from build123d import *

# Parameters (mm, degrees)
SKETCH1_R                       = 8
BOSS_EXTRUDE1_DEPTH             = 10
SKETCH2_R                       = 12.6
BOSS_EXTRUDE2_DEPTH             = 3
SKETCH4_R                       = 1.5
CUT_EXTRUDE4_DEPTH              = 13
SKETCH3_R                       = 12.6
BOSS_EXTRUDE4_DEPTH             = 5
SKETCH5_R                       = 2.1
CUT_EXTRUDE5_DEPTH              = 19
SKETCH6_W                       = 1
SKETCH6_H                       = 4.89371283
BOSS_EXTRUDE5_DEPTH             = 8
TAP_DRILL_FOR_M2X0_4_TAP1_D     = 1.6
TAP_DRILL_FOR_M2X0_4_TAP1_DEPTH = 16
TAP_DRILL_FOR_M2X0_4_TAP1_TIP   = 0.480688495
SKETCH16_R                      = 15.644014
BOSS_EXTRUDE6_DEPTH             = 5
SKETCH17_R                      = 2.1
CUT_EXTRUDE6_DEPTH              = 5
SKETCH18_R                      = 1.1
CUT_EXTRUDE9_DEPTH              = 9.0000001
SKETCH19_R                      = 1.1
CUT_EXTRUDE10_DEPTH             = 10


with BuildPart() as part:
    # Sketch1 → Boss-Extrude1 (new body)
    with BuildSketch(Plane(origin=(0, 0, 0), x_dir=(1, 0, 0), z_dir=(0, 1, 0))):
        Circle(SKETCH1_R)
    extrude(amount=BOSS_EXTRUDE1_DEPTH)

    # Sketch2 → Boss-Extrude2 (add)
    with BuildSketch(Plane.XZ):
        Circle(SKETCH2_R)
    extrude(amount=BOSS_EXTRUDE2_DEPTH)

    # Sketch4 → Cut-Extrude4 (cut)
    with BuildSketch(Plane(origin=(0, 10, 0), x_dir=(1, 0, 0), z_dir=(0, 1, 0))):
        Circle(SKETCH4_R)
    extrude(amount=-CUT_EXTRUDE4_DEPTH, mode=Mode.SUBTRACT)

    # Sketch3 → Boss-Extrude4 (add)
    with BuildSketch(Plane(origin=(0, 10, 0), x_dir=(1, 0, 0), z_dir=(0, 1, 0))):
        Circle(SKETCH3_R)
    extrude(amount=BOSS_EXTRUDE4_DEPTH)

    # Sketch5 → Cut-Extrude5 (cut, through all)
    with BuildSketch(Plane(origin=(0, 15, 0), x_dir=(1, 0, 0), z_dir=(0, 1, 0))):
        Circle(SKETCH5_R)
    extrude(amount=-CUT_EXTRUDE5_DEPTH, mode=Mode.SUBTRACT)

    # Sketch6 → Boss-Extrude5 (add)
    with BuildSketch(Plane(origin=(0, 15, 0), x_dir=(1, 0, 0), z_dir=(0, 1, 0))):
        with Locations((-2.1, 0)):
            Rectangle(SKETCH6_W, SKETCH6_H)
    extrude(amount=-BOSS_EXTRUDE5_DEPTH)

    # Tap Drill for M2x0.4 Tap1
    with Locations(Plane.ZY.offset(12.6)):
        with Locations((0, 12.5)):
            Hole(TAP_DRILL_FOR_M2X0_4_TAP1_D / 2, depth=TAP_DRILL_FOR_M2X0_4_TAP1_DEPTH)
            with Locations((0, 0, -(TAP_DRILL_FOR_M2X0_4_TAP1_DEPTH + TAP_DRILL_FOR_M2X0_4_TAP1_TIP / 2))):  # 118° drill point
                Cone(0, TAP_DRILL_FOR_M2X0_4_TAP1_D / 2, TAP_DRILL_FOR_M2X0_4_TAP1_TIP, mode=Mode.SUBTRACT)

    # Sketch16 → Boss-Extrude6 (add)
    with BuildSketch(Plane(origin=(0, -3, 0), x_dir=(-1, 0, 0), z_dir=(0, -1, 0))):
        Circle(SKETCH16_R)
    extrude(amount=BOSS_EXTRUDE6_DEPTH)

    # Sketch17 → Cut-Extrude6 (cut)
    with BuildSketch(Plane(origin=(0, -8, 0), x_dir=(-1, 0, 0), z_dir=(0, -1, 0))):
        Circle(SKETCH17_R)
    extrude(amount=-CUT_EXTRUDE6_DEPTH, mode=Mode.SUBTRACT)

    # Sketch18 → Cut-Extrude9 (cut, through all)
    with BuildSketch(Plane(origin=(0, 0, 0), x_dir=(1, 0, 0), z_dir=(0, 1, 0))):
        with Locations((-9.4, 0)):
            Circle(SKETCH18_R)
    extrude(amount=-CUT_EXTRUDE9_DEPTH, mode=Mode.SUBTRACT)

    # Sketch19 → Cut-Extrude10 (cut)
    with BuildSketch(Plane(origin=(0, 10, 0), x_dir=(-1, 0, 0), z_dir=(0, -1, 0))):
        with Locations((-9.4, 0)):
            Circle(SKETCH19_R)
    extrude(amount=-CUT_EXTRUDE10_DEPTH, mode=Mode.SUBTRACT)


solid = part.part
Build history of the part. All positions in model axes, mm. A direction names the side the tool comes from. Round coordinates to 2 decimals unless told otherwise and drop trailing zeros. Write each loop counter-clockwise with the first axis right and the second up, starting at its lowest first coordinate (ties: lowest second). Pieces come first, ordered by that corner, then holes. Notation, with made-up numbers: M -37.75,-36.75 L -14.75,-36.75 A26 cw -14.75,-16.75 Z; hole C 29,5 d6. An arc over 180 degrees is marked long. Answer in a Markdown table with one row per item.
1. Saw through at A-A (x = -10). List the corners of the cut face in (y, z).
Geometry check:
| item | result |
|---|---|
| outline | M -8,-12.03 L -3,-12.03 L -3,-7.67 L 0,-7.67 L 0,-0.92 L -8,-0.92 Z; M -8,0.92 L 0,0.92 L 0,7.67 L -3,7.67 L -3,12.03 L -8,12.03 Z; M 10,-7.67 L 15,-7.67 L 15,7.67 L 10,7.67 Z; hole C 12.5,0 d1.6 |
2. Probe L1, parallel to Z at x = 0, y = 4.75; L2, parallel to Y at x = 11, z = -4; L3, parallel to Z at x = 0, y = 10.5. List the from-to ranges inside material, lowest first. Write a range as [from, to].
Geometry check:
| item | result |
|---|---|
| L1 | [-8, -2.1], [2.1, 8] |
| L2 | [-8, 0], [10, 15] |
| L3 | [-12.6, -2.1], [2.1, 12.6] |
3. Flat gauge pins, fed straight in: P1, Ø1.8, axis at y = 12.5, z = 0, coming from the -X side; P2, Ø4, axis at x = -9, y = 4.5, coming from the +Z side; P3, Ø8, axis at y = -4.5, z = -9.5, coming from the +X side. Where does each tip first touch, or does it go through?
Geometry check:
| item | result |
|---|---|
| P1 | x = -12.6 |
| P2 | z = 3.87 |
| P3 | x = 14.65 |
4. Saw through at D-D (x = 9.4). List the corners of the cut face in (y, z) (3 decimals), and give its area (3 significant figures).
Geometry check:
| item | result |
|---|---|
| outline | M -8,-12.505 L -3,-12.505 L -3,-8.39 L 0,-8.39 L 0,8.39 L -3,8.39 L -3,12.505 L -8,12.505 Z; M 10,-8.39 L 15,-8.39 L 15,-1.1 L 10,-1.1 Z; M 10,1.1 L 15,1.1 L 15,8.39 L 10,8.39 Z |
| area | 248 mm2 |
5. Saw through at C-C (y = -1.5). List the corners of the cut face in (x, z), and give its area (3 significant figures).
Geometry check:
| item | result |
|---|---|
| outline | C 0,0 d25.2; hole C -9.4,0 d2.2; hole C 0,0 d4.2 |
| area | 481 mm2 |
6. Saw through at B-B (x = 0). List the corners of the cut face in (y, z).
Geometry check:
| item | result |
|---|---|
| outline | M -8,-15.64 L -3,-15.64 L -3,-12.6 L 0,-12.6 L 0,-8 L 10,-8 L 10,-12.6 L 15,-12.6 L 15,-2.1 L -8,-2.1 Z; M -8,2.1 L 15,2.1 L 15,12.6 L 10,12.6 L 10,8 L 0,8 L 0,12.6 L -3,12.6 L -3,15.64 L -8,15.64 Z |
7. Mould opens along Y. For faces 1 (the face through (2.7, 12.5, 0.8)), 2 (the face through (-10.27, -3.94, 0.67)), 3 (the face through (0, 15, 3)) say: +Y half, -Y half, draft (parallel to the pull), parting line (faces both ways), or undercut.
Geometry check:
| item | result |
|---|---|
| face 1 | undercut |
| face 2 | draft |
| face 3 | +Y half |
8. Which spindle directions (+Z, -Z, +X, -X, +Y, -Y) get a long thin tool onto all of the face, cutting with end or side? Do faces 4 (the face through (-1.6, 11, 0)), 5 (the face through (-7.02, 12.01, 0.63)), 6 (the face through (-9.999, -1.479, -7.667)). Say none if no direction does.
Geometry check:
| item | result |
|---|---|
| face 4 | +Y, -Y |
| face 5 | -X |
| face 6 | +Y |
